from build123d import *

# Parameters (mm, degrees)
SKETCH_1_R           = 3
SKETCH_1_R_2         = 2.5
EXTRUDE_1_DEPTH      = 6
SKETCH_1_8_R         = 2.5
EXTRUDE_2_DEPTH      = 11.5
SKETCH_1_9_R         = 9
EXTRUDE_3_DEPTH      = 3
SKETCH_6_W           = 0.15
SKETCH_6_H           = 0.5
HOLE_WIZARD_M2_5_1_D = 2.05


with BuildPart() as part:
    # 草图1 → 凸台-拉伸1 (new body)
    with BuildSketch(Plane(origin=(0, 0, 0), x_dir=(1, 0, 0), z_dir=(0, 1, 0))):
        Circle(SKETCH_1_R)
        Circle(SKETCH_1_R_2, mode=Mode.SUBTRACT)
    extrude(amount=EXTRUDE_1_DEPTH)

    # 草图1<8> → 凸台-拉伸2 (add)
    with BuildSketch(Plane(origin=(0, 0, 0), x_dir=(1, 0, 0), z_dir=(0, 1, 0))):
        Circle(SKETCH_1_8_R)
    extrude(amount=EXTRUDE_2_DEPTH)

    # 草图1<9> → 凸台-拉伸3 (add)
    with BuildSketch(Plane(origin=(0, 0, 0), x_dir=(1, 0, 0), z_dir=(0, 1, 0))):
        Circle(SKETCH_1_9_R)
    extrude(amount=-EXTRUDE_3_DEPTH)

    # 草图6 → 切除-旋转1 (revolve, cut)
    with BuildSketch(Plane(origin=(0, 0, 0), x_dir=(0, 0, -1), z_dir=(1, 0, 0))):
        with Locations((-2.425, 10.25)):
            Rectangle(SKETCH_6_W, SKETCH_6_H)
    revolve(axis=Axis((0, 9, 0), (0, -1, 0)), mode=Mode.SUBTRACT)

    # M2.5 螺纹孔1 (through all)
    with Locations(Plane(origin=(0, 0, 0), x_dir=(1, 0, 0), z_dir=(0, 1, 0))):
        with Locations((-5.196152423, -3), (0, 6), (5.196152423, -3)):
            Hole(HOLE_WIZARD_M2_5_1_D / 2)


solid = part.part
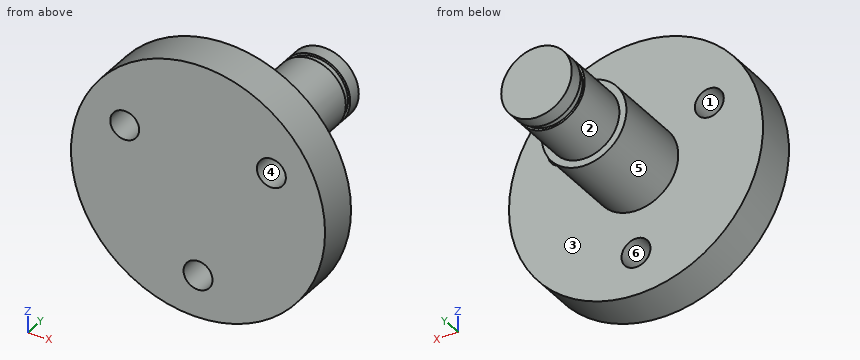
Check sheet for the modelled part. Datum: model origin and axes. Units: mm. Face numbers are marked on the shaded views. A direction names the side the tool comes from. Round coordinates to 2 decimals unless told otherwise and drop trailing zeros. Order: outer loops, then holes, each group sorted by start corner. A loop starts at its lowest first (then second) coordinate and runs counter-clockwise, first axis right, second up.
Q1. Cross-section at D-D, the plane y = -2. Enter the section's corners in (x, z) (3 decimals), plus the area to 3 significant figures.
Filled sheet:
outline: circle Ø18 at (0, 0); hole circle Ø2.05 at (-5.196, 3); hole circle Ø2.05 at (0, -6); hole circle Ø2.05 at (5.196, 3)
area: 245 mm2
Q2. Scan lines: L1, parallel to Z at x = 0, y = -1.9 (3 decimals); L2, parallel to Y at x = 6, z = -2.5; L3, parallel to X at y = -0.75, z = -0.25. Record each from-to range of solid material in increasing order.
Filled sheet:
L1: z = -9 to -7.025, -4.975 to 9
L2: y = -3 to 0
L3: x = -9 to 9
Q3. Depth check by flat-ended pin: P1, Ø5.5, axis at x = 3.5, z = 3, coming from the +Y side; P2, Ø6, axis at x = 5, y = 1, coming from the -Z side; P3, Ø2.5, axis at x = 0, z = -6, coming from the +Y side; P4, Ø8, axis at x = -5, y = 4.5, coming from the -Z side. Enter the tip coordinate at first touch or a pass-through.
Filled sheet:
P1: stops at y = 11.5
P2: stops at z = -8.73
P3: stops at y = 0
P4: stops at z = -2.83
Q4. Cross-section at A-A, the plane x = 0. Enter the section's corners in (y, z) (3 decimals), plus the area to 3 significant figures.
Filled sheet:
outline: (-3, -9) - (0, -9) - (0, -7.025) - (-3, -7.025) - close; (-3, -4.975) - (0, -4.975) - (0, -3) - (6, -3) - (6, -2.5) - (10, -2.5) - (10, -2.35) - (10.5, -2.35) - (10.5, -2.5) - (11.5, -2.5) - (11.5, 2.5) - (10.5, 2.5) - (10.5, 2.35) - (10, 2.35) - (10, 2.5) - (6, 2.5) - (6, 3) - (0, 3) - (0, 9) - (-3, 9) - close
area: 111 mm2
Q5. Set-up check for the marked faces 5 and 6: record each of +Z, -Z, +X, -X, +Y, -Y from which the full face is reachable in a straight line by a thin tool's end or side.
Filled sheet:
face 5: +Y
face 6: +Y, -Y
Q6. Cross-section at C-C, the plane z = -6. Enter the section's corners in (x, y) (3 decimals), plus the area to 3 significant figures.
Filled sheet:
outline: (-6.708, -3) - (-1.025, -3) - (-1.025, 0) - (-6.708, 0) - close; (1.025, -3) - (6.708, -3) - (6.708, 0) - (1.025, 0) - close
area: 34.1 mm2
Q7. Cross-section at B-B, the plane z = 0. Enter the section's corners in (x, y), plus the area to 3 significant figures.
Filled sheet:
outline: (-9, -3) - (9, -3) - (9, 0) - (3, 0) - (3, 6) - (2.5, 6) - (2.5, 10) - (2.35, 10) - (2.35, 10.5) - (2.5, 10.5) - (2.5, 11.5) - (-2.5, 11.5) - (-2.5, 10.5) - (-2.35, 10.5) - (-2.35, 10) - (-2.5, 10) - (-2.5, 6) - (-3, 6) - (-3, 0) - (-9, 0) - close
area: 117 mm2
Q8. Draft check along Z on the marked faces 1, 2, 3 and 4. Enter one of: pulls with the +Z half, pulls with the -Z half, needs draft (parallel to the pull), parting line crosses it, or undercut.
Filled sheet:
face 1: undercut
face 2: parting line crosses it
face 3: needs draft
face 4: undercut
